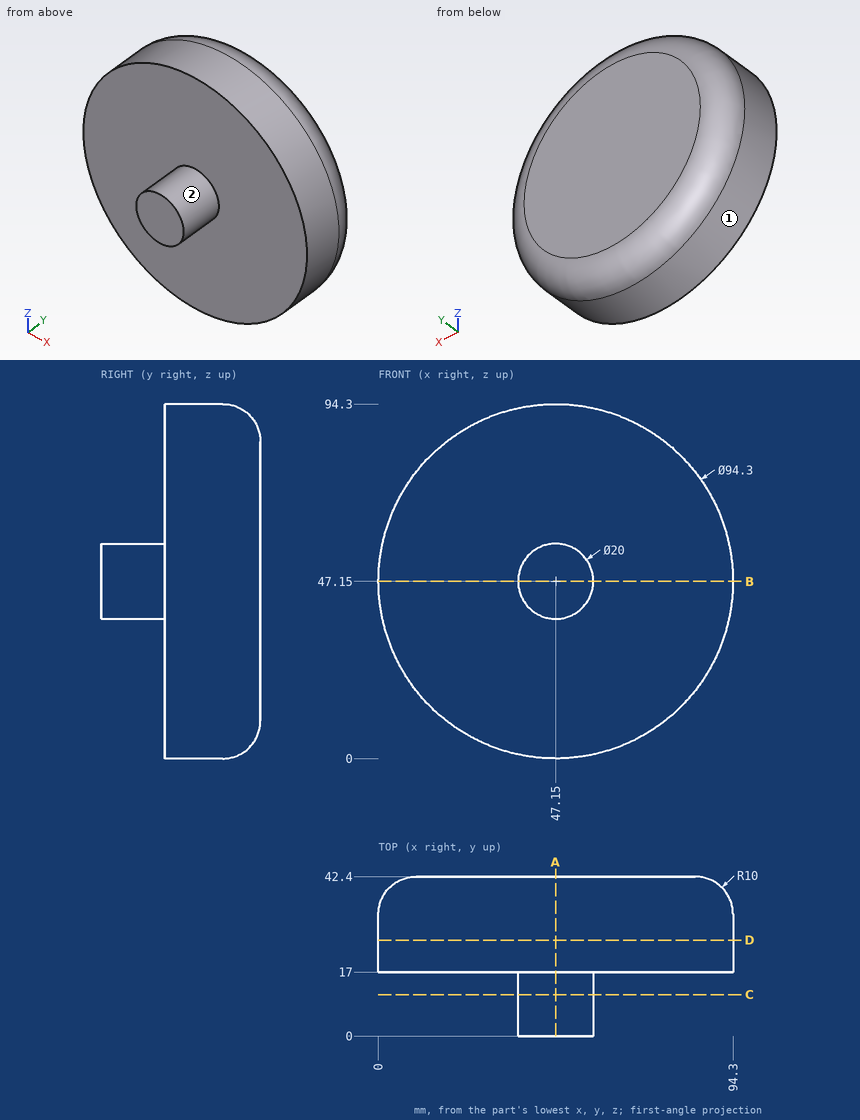
Geometry check sheet. Reference: drawing and pictorial views, mm from the part's lowest x, y, z. A direction names the side the tool comes from. Give positions to 0.01 mm unless a question says otherwise; leave off trailing zeros. Write each loop counter-clockwise with the first axis right and the second up, starting at its lowest first coordinate (ties: lowest second). Pieces come first, ordered by that corner, then holes.
Item 1: Access from +Z, -Z, +X, -X, +Y, -Y to the whole of each face (thin tool, end or side, straight path). Record for the marked faces 1 and 2.
Item 2: Cross-section at C-C (y = 11). Enter the section's corners in (x, z), and give its area (3 significant figures).
Item 3: Cross-section at A-A (x = 47.15). Enter the section's corners in (y, z).
Item 4: Cross-section at B-B (z = 47.15). Enter the section's corners in (x, y), and give its area (3 significant figures).
Item 5: Scan lines: L1, parallel to Y at x = 62, z = 57; L2, parallel to Y at x = 31, z = 84; L3, parallel to Z at x = 61.5, y = 23.5. Record each from-to range of solid material in increasing order.
Item 6: Cross-section at D-D (y = 25.5). Enter the section's corners in (x, z), and give its area (3 significant figures).
Item 7: Gauge pin test, flat ends, axial feed: pin 1 (10 mm diameter, centred on x = 45, y = 35.5, fed in from +Z); pin 2 (5 mm diameter, centred on x = 58.5, z = 12.5, fed in from -Y); pin 3 (2 mm diameter, centred on x = 28, y = 26.5, fed in from -Z). Record the tip position at first contact, or that the pin passes through.
Report:
1. face 1: +Y, -Y
1. face 2: -Y
2. outline: circle Ø20 at (47.15, 47.15)
2. area: 314 mm2
3. outline: (0, 37.15) - (17, 37.15) - (17, 0) - (32.4, 0) arc R10 ccw to (42.4, 10) - (42.4, 84.3) arc R10 ccw to (32.4, 94.3) - (17, 94.3) - (17, 57.15) - (0, 57.15) - close
4. outline: (0, 17) - (37.15, 17) - (37.15, 0) - (57.15, 0) - (57.15, 17) - (94.3, 17) - (94.3, 32.4) arc R10 ccw to (84.3, 42.4) - (10, 42.4) arc R10 ccw to (0, 32.4) - close
4. area: 2,690 mm2
5. L1: y = 17 to 42.4
5. L2: y = 17 to 41.91
5. L3: z = 2.24 to 92.06
6. outline: circle Ø94.3 at (47.15, 47.15)
6. area: 6,980 mm2
7. pin 1: stops at z = 94.3
7. pin 2: stops at y = 17
7. pin 3: stops at z = 3.63
